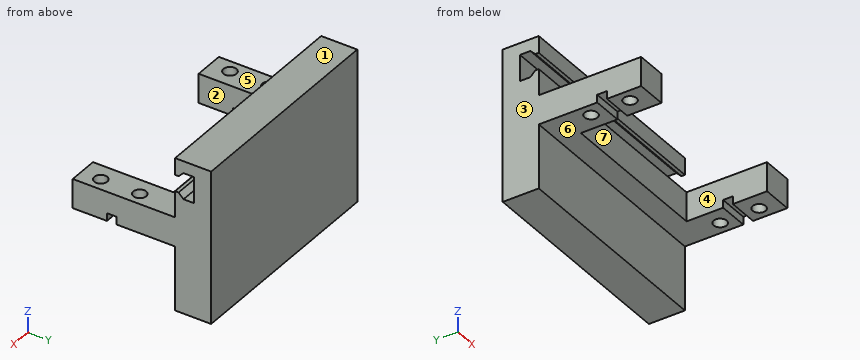
```python
from build123d import *

# Parameters (mm, degrees)
BOSS_EXTRUDE1_DEPTH = 56
BOSS_EXTRUDE2_DEPTH = 56
CUT_EXTRUDE1_REACH  = 74.056
SKETCH6_R           = 1.672
CUT_EXTRUDE4_DEPTH  = 7.5


with BuildPart() as part:
    # Sketch2 → Boss-Extrude1 (new body)
    with BuildSketch(Plane(origin=(0, 0, 0), x_dir=(0, 0, -1), z_dir=(1, 0, 0))):
        Polygon((-39.250001311, 38.490001112), (-39.250001311, 29.240000993), (-34.930501133, 29.240000993), (-34.930501133, 30.129000545), (-36.200501025, 31.399000436), (-36.200501025, 34.065999091), (-29.469501227, 34.065999091), (-29.469501227, 31.399000436), (-30.739501119, 30.129000545), (-30.739501119, 29.240000993), (-0.03858842, 29.240000993), (-0.03858842, 38.490001112), align=None)
    extrude(amount=BOSS_EXTRUDE1_DEPTH)

    # Sketch3 → Boss-Extrude2 (add)
    with BuildSketch(Plane(origin=(56, 0, 0), x_dir=(0, 0, -1), z_dir=(1, 0, 0))):
        Polygon((-18.510001311, 29.240000993), (-24.010001311, 29.240000993), (-24.010001311, 2.969290993), (-16.510001311, 2.969290993), (-16.510001311, 11.750000993), (-18.510001311, 11.750000993), (-18.510001311, 14.250000993), (-16.510001311, 14.250000993), (-16.510001311, 29.240000993), align=None)
    extrude(amount=-BOSS_EXTRUDE2_DEPTH)

    # Cut-Extrude1: up to this face of the body (flat: up to its plane)
    cut_extrude1_end = Plane(part.part.faces().sort_by_distance((28, 21.745000993, 16.510001311))[0])
    # Sketch4 → Cut-Extrude1 (cut, up to the picked face)
    with BuildSketch(Plane.XY.offset(24.010001311), mode=Mode.PRIVATE) as cut_extrude1_sk1:
        Polygon((48.254, 23.631000993), (26.180665343, 23.631000993), (7.746, 23.631000993), (7.746, 20.223656135), (7.746, 7.540175529), (7.746, 2.969290993), (48.254, 2.969290993), (48.254, 20.898309359), align=None)
    cut_extrude1_tool1 = split(extrude(cut_extrude1_sk1.sketch, amount=-CUT_EXTRUDE1_REACH, mode=Mode.PRIVATE), bisect_by=cut_extrude1_end, keep=Keep.BOTH, mode=Mode.PRIVATE)
    add(cut_extrude1_tool1.solids().sort_by(Axis((28, 13.300146, 24.010001), (0, 0, -1)))[0], mode=Mode.SUBTRACT)

    # Sketch6 → Cut-Extrude4 (cut)
    with BuildSketch(Plane.XY.offset(24.010001311)):
        with Locations((3.25, 18.000000993)):
            Circle(SKETCH6_R)
        with Locations((3.25, 8.000000993)):
            Circle(SKETCH6_R)
        with Locations((52.75, 18.000000993)):
            Circle(SKETCH6_R)
        with Locations((52.75, 8.000000993)):
            Circle(SKETCH6_R)
    extrude(amount=-CUT_EXTRUDE4_DEPTH, mode=Mode.SUBTRACT)


solid = part.part
```
Work out the finished part from the listing and answer in its coordinate system (mm). Face numbers are marked on the shaded views. A direction names the side the tool comes from. Coordinates: 2 decimals unless noted, no trailing zeros. Loops run counter-clockwise (first coordinate to the right, second up) from the corner with the lowest first, then second, coordinate; pieces in that order, holes last. Notation, with made-up numbers: M -33.75,54.5 L -6.75,54.5 A25 cw -6.75,79.5 Z; hole C 32.25,75 d8. An arc over 180 degrees is marked long. Use CSV: the item, a comma, the result in double quotes. Start each with the question number.
(1) For the marked faces 5, 6 and 7, determine the directions among +Z, -Z, +X, -X, +Y, -Y from which every point of the face is accessible in a straight line to the end or side of a thin tool.
(2) Given pin 1 Ø4 at (x, y) = (3.25, 18) entering from -Z; pin 2 Ø2 at (x, z) = (34.5, 21.5) entering from -Y; pin 3 Ø0.8 at (x, y) = (5, 12.5) entering from -Z, each flat-ended and moving along its own axis, determine where each tip first touches the part or whether it passes through.
(3) Find section D-D, the plane x = 39.5. Give the vertices of the cut face in (y, z), then the cut area to 3 significant figures.
(4) Find section C-C, the plane y = 22.5. Give the vertices of the cut face in (x, z).
(5) Find section A-A, the plane y = 8. Give the vertices of the cut face in (x, z), then the cut area to 3 significant figures.
(6) Find section B-B, the plane x = 3.25. Give the vertices of the cut face in (y, z), then the cut area to 3 significant figures.
(7) For a pull along X with two mould halves and no side action, classify the marked faces 1, 2, 3 and 4 as +X half, -X half, draft (parallel to the pull), parting line (faces both ways), or undercut.
(8) Consider line 1 (Y direction, x = 52.75, z = 19); line 2 (X direction, y = 20.5, z = 19.5); line 3 (Z direction, x = 49, y = 33.5). Determine where each line is inside the solid, lowest interval first.
Recorded:
1,face 5,"+Z, +X, -X, -Y"
1,face 6,"-Z, +X, -X, -Y"
1,face 7,"+Z, -Z, -Y"
2,pin 1,"stops at z = 16.51"
2,pin 2,"stops at y = 23.63"
2,pin 3,"stops at z = 18.51"
3,outline,"M 23.63,16.51 L 29.24,16.51 L 29.24,0.04 L 38.49,0.04 L 38.49,39.25 L 29.24,39.25 L 29.24,34.93 L 30.13,34.93 L 31.4,36.2 L 34.07,36.2 L 34.07,29.47 L 31.4,29.47 L 30.13,30.74 L 29.24,30.74 L 29.24,24.01 L 23.63,24.01 Z"
3,area,"376 mm^2"
4,outline,"M 0,16.51 L 7.75,16.51 L 7.75,24.01 L 0,24.01 Z; M 48.25,16.51 L 56,16.51 L 56,24.01 L 48.25,24.01 Z"
5,outline,"M 0,16.51 L 1.58,16.51 L 1.58,24.01 L 0,24.01 Z; M 4.92,16.51 L 7.75,16.51 L 7.75,24.01 L 4.92,24.01 Z; M 48.25,16.51 L 51.08,16.51 L 51.08,24.01 L 48.25,24.01 Z; M 54.42,16.51 L 56,16.51 L 56,24.01 L 54.42,24.01 Z"
5,area,"66.0 mm^2"
6,outline,"M 2.97,16.51 L 6.33,16.51 L 6.33,24.01 L 2.97,24.01 Z; M 9.67,16.51 L 11.75,16.51 L 11.75,18.51 L 14.25,18.51 L 14.25,16.51 L 16.33,16.51 L 16.33,24.01 L 9.67,24.01 Z; M 19.67,16.51 L 29.24,16.51 L 29.24,0.04 L 38.49,0.04 L 38.49,39.25 L 29.24,39.25 L 29.24,34.93 L 30.13,34.93 L 31.4,36.2 L 34.07,36.2 L 34.07,29.47 L 31.4,29.47 L 30.13,30.74 L 29.24,30.74 L 29.24,24.01 L 19.67,24.01 Z"
6,area,"476 mm^2"
7,face 1,"draft"
7,face 2,"undercut"
7,face 3,"-X half"
7,face 4,"undercut"
8,line 1,"y = 2.97 to 6.33, 9.67 to 16.33, 19.67 to 38.49"
8,line 2,"x = 0 to 7.75, 48.25 to 56"
8,line 3,"z = 0.04 to 29.47, 36.2 to 39.25"
